```python
from build123d import *

# Parameters (mm, degrees)
SALIENTE_EXTRUIR1_DEPTH = 0.8
CORTAR_EXTRUIR1_REACH   = 182
CROQUIS3_R              = 1.585
CORTAR_EXTRUIR2_DEPTH   = 0.8
CORTAR_EXTRUIR3_REACH   = 2.8
CROQUIS4_R              = 1.585
CORTAR_EXTRUIR4_REACH   = 2.8
CROQUIS6_R              = 1.585
CROQUIS7_R              = 1.585
CORTAR_EXTRUIR5_DEPTH   = 0.8


with BuildPart() as part:
    # Croquis1 → Saliente-Extruir1 (new body)
    with BuildSketch(Plane(origin=(0, 0, 0), x_dir=(1, 0, 0), z_dir=(0, 1, 0))):
        Polygon((-62.5, 90), (-62.5, 27.08), (-90, 27.08), (-90, -90), (90, -90), (90, 27.08), (62.5, 27.08), (62.5, 90), align=None)
    extrude(amount=SALIENTE_EXTRUIR1_DEPTH)

    # Croquis2 → Cortar-Extruir1 (cut, up to next)
    with BuildSketch(Plane.ZY.offset(90), mode=Mode.PRIVATE) as cortar_extruir1_sk1:
        Polygon((90, 0), (88.614359354, 0.8), (90, 0.8), align=None)
    cortar_extruir1_tool1 = extrude(cortar_extruir1_sk1.sketch, amount=-CORTAR_EXTRUIR1_REACH, mode=Mode.PRIVATE) & part.part
    add(cortar_extruir1_tool1.solids().sort_by_distance((-90, 0.533333, 89.53812))[0], mode=Mode.SUBTRACT)

    # Croquis3 → Cortar-Extruir2 (cut)
    with BuildSketch(Plane(origin=(0, 0.8, 0), x_dir=(1, 0, 0), z_dir=(0, 1, 0))):
        with Locations((74, -24.279339937)):
            Circle(CROQUIS3_R)
    cortar_extruir2 = extrude(amount=-CORTAR_EXTRUIR2_DEPTH, mode=Mode.SUBTRACT)

    # Simetría1: Cortar-Extruir2 across plane
    add(cortar_extruir2.mirror(Plane(origin=(0, 0, 0), x_dir=(0, 0, 1), z_dir=(1, 0, 0))), mode=Mode.SUBTRACT)

    # Croquis4 → Cortar-Extruir3 (cut, up to next)
    with BuildSketch(Plane(origin=(0, 0.8, 0), x_dir=(1, 0, 0), z_dir=(0, 1, 0)), mode=Mode.PRIVATE) as cortar_extruir3_sk1:
        with Locations((-56.5, 36.505640646)):
            Circle(CROQUIS4_R)
    cortar_extruir3_tool1 = extrude(cortar_extruir3_sk1.sketch, amount=-CORTAR_EXTRUIR3_REACH, mode=Mode.PRIVATE) & part.part
    add(cortar_extruir3_tool1.solids().sort_by_distance((-56.5, 0.8, -36.505641))[0], mode=Mode.SUBTRACT)
    # Croquis4 → Cortar-Extruir3 (cut, up to next)
    with BuildSketch(Plane(origin=(0, 0.8, 0), x_dir=(1, 0, 0), z_dir=(0, 1, 0)), mode=Mode.PRIVATE) as cortar_extruir3_sk2:
        with Locations((-15.5, 36.505640646)):
            Circle(CROQUIS4_R)
    cortar_extruir3_tool2 = extrude(cortar_extruir3_sk2.sketch, amount=-CORTAR_EXTRUIR3_REACH, mode=Mode.PRIVATE) & part.part
    add(cortar_extruir3_tool2.solids().sort_by_distance((-15.5, 0.8, -36.505641))[0], mode=Mode.SUBTRACT)
    # Croquis4 → Cortar-Extruir3 (cut, up to next)
    with BuildSketch(Plane(origin=(0, 0.8, 0), x_dir=(1, 0, 0), z_dir=(0, 1, 0)), mode=Mode.PRIVATE) as cortar_extruir3_sk3:
        with Locations((-15.5, 85.005640646)):
            Circle(CROQUIS4_R)
    cortar_extruir3_tool3 = extrude(cortar_extruir3_sk3.sketch, amount=-CORTAR_EXTRUIR3_REACH, mode=Mode.PRIVATE) & part.part
    add(cortar_extruir3_tool3.solids().sort_by_distance((-15.5, 0.8, -85.005641))[0], mode=Mode.SUBTRACT)
    # Croquis4 → Cortar-Extruir3 (cut, up to next)
    with BuildSketch(Plane(origin=(0, 0.8, 0), x_dir=(1, 0, 0), z_dir=(0, 1, 0)), mode=Mode.PRIVATE) as cortar_extruir3_sk4:
        with Locations((-56.5, 85.005640646)):
            Circle(CROQUIS4_R)
    cortar_extruir3_tool4 = extrude(cortar_extruir3_sk4.sketch, amount=-CORTAR_EXTRUIR3_REACH, mode=Mode.PRIVATE) & part.part
    add(cortar_extruir3_tool4.solids().sort_by_distance((-56.5, 0.8, -85.005641))[0], mode=Mode.SUBTRACT)

    # Croquis6 → Cortar-Extruir4 (cut, up to next)
    with BuildSketch(Plane(origin=(0, 0.8, 0), x_dir=(1, 0, 0), z_dir=(0, 1, 0)), mode=Mode.PRIVATE) as cortar_extruir4_sk1:
        with Locations((56.5, 85.005640646)):
            Circle(CROQUIS6_R)
    cortar_extruir4_tool1 = extrude(cortar_extruir4_sk1.sketch, amount=-CORTAR_EXTRUIR4_REACH, mode=Mode.PRIVATE) & part.part
    add(cortar_extruir4_tool1.solids().sort_by_distance((56.5, 0.8, -85.005641))[0], mode=Mode.SUBTRACT)
    # Croquis6 → Cortar-Extruir4 (cut, up to next)
    with BuildSketch(Plane(origin=(0, 0.8, 0), x_dir=(1, 0, 0), z_dir=(0, 1, 0)), mode=Mode.PRIVATE) as cortar_extruir4_sk2:
        with Locations((15.5, 85.005640646)):
            Circle(CROQUIS6_R)
    cortar_extruir4_tool2 = extrude(cortar_extruir4_sk2.sketch, amount=-CORTAR_EXTRUIR4_REACH, mode=Mode.PRIVATE) & part.part
    add(cortar_extruir4_tool2.solids().sort_by_distance((15.5, 0.8, -85.005641))[0], mode=Mode.SUBTRACT)
    # Croquis6 → Cortar-Extruir4 (cut, up to next)
    with BuildSketch(Plane(origin=(0, 0.8, 0), x_dir=(1, 0, 0), z_dir=(0, 1, 0)), mode=Mode.PRIVATE) as cortar_extruir4_sk3:
        with Locations((15.5, 36.505640646)):
            Circle(CROQUIS6_R)
    cortar_extruir4_tool3 = extrude(cortar_extruir4_sk3.sketch, amount=-CORTAR_EXTRUIR4_REACH, mode=Mode.PRIVATE) & part.part
    add(cortar_extruir4_tool3.solids().sort_by_distance((15.5, 0.8, -36.505641))[0], mode=Mode.SUBTRACT)
    # Croquis6 → Cortar-Extruir4 (cut, up to next)
    with BuildSketch(Plane(origin=(0, 0.8, 0), x_dir=(1, 0, 0), z_dir=(0, 1, 0)), mode=Mode.PRIVATE) as cortar_extruir4_sk4:
        with Locations((56.5, 36.505640646)):
            Circle(CROQUIS6_R)
    cortar_extruir4_tool4 = extrude(cortar_extruir4_sk4.sketch, amount=-CORTAR_EXTRUIR4_REACH, mode=Mode.PRIVATE) & part.part
    add(cortar_extruir4_tool4.solids().sort_by_distance((56.5, 0.8, -36.505641))[0], mode=Mode.SUBTRACT)

    # Croquis7 → Cortar-Extruir5 (cut)
    with BuildSketch(Plane(origin=(0, 0.8, 0), x_dir=(1, 0, 0), z_dir=(0, 1, 0))):
        with Locations((-20, 85.005640646)):
            Circle(CROQUIS7_R)
        with Locations((-47.5, 85.005640646)):
            Circle(CROQUIS7_R)
        with Locations((-47.5, 55.005640646)):
            Circle(CROQUIS7_R)
        with Locations((-20, 55.005640646)):
            Circle(CROQUIS7_R)
    cortar_extruir5 = extrude(amount=-CORTAR_EXTRUIR5_DEPTH, mode=Mode.SUBTRACT)

    # Simetría2: Cortar-Extruir5 across plane
    add(cortar_extruir5.mirror(Plane(origin=(0, 0, 0), x_dir=(0, 0, 1), z_dir=(1, 0, 0))), mode=Mode.SUBTRACT)


solid = part.part
```
Geometry: final body of the model. Coordinates: model frame, mm. Coordinates: 2 decimals unless noted, no trailing zeros. Order: outer loops, then holes, each group sorted by start corner. A loop starts at its lowest first (then second) coordinate and runs counter-clockwise, first axis right, second up. Notation, with made-up numbers: (47, 44) - (78, 44) arc R8 cw to (78, 56) - close; hole circle Ø10 at (35.5, 38.25). An arc over 180 degrees is marked (long way). Write each question's results on one line, items separated by ' | '.
1) Section A-A, the plane y = 0.65. State how many separate pieces and enclosed holes the cut face has, plus the area to 3 significant figures.
Results list:
separate pieces: 1 | enclosed holes: 18 | area: 28,600 mm^2
2) Section B-B, the plane z = -67.5. Return loops of the section in (x, y).
Results list:
outline: (-62.5, 0) - (62.5, 0) - (62.5, 0.8) - (-62.5, 0.8) - close
3) Line query: line 1 (Z direction, x = -56.5, y = 0.25); line 2 (Z direction, x = 15.5, y = 0.4); line 3 (X direction, y = 0.7, z = -40.5). Output: solid intervals per line, ascending. Write a range as from..to.
Results list:
line 1: -90..-86.59, -83.42..-38.09, -34.92..89.57 | line 2: -90..-86.59, -83.42..-38.09, -34.92..89.31 | line 3: -62.5..62.5
4) Pin query (flat end, axial travel): pin 1 (2.5 mm diameter, centred on x = -47.5, z = -55.01, fed in from +Y). Return the tip coordinate at first contact, or that it passes through.
Results list:
pin 1: through
